```python
from build123d import *

# Parameters (mm, degrees)
SKETCH1_W           = 120
SKETCH1_H           = 31
BOSS_EXTRUDE1_DEPTH = 10
SKETCH4_R           = 3
BOSS_EXTRUDE2_DEPTH = 30
FILLET1_R           = 2


with BuildPart() as part:
    # Sketch1 → Boss-Extrude1 (new body, symmetric)
    with BuildSketch(Plane(origin=(0, 0, 0), x_dir=(1, 0, 0), z_dir=(0, 1, 0))):
        Rectangle(SKETCH1_W, SKETCH1_H)
    extrude(amount=BOSS_EXTRUDE1_DEPTH, both=True)

    # Sketch4 → Boss-Extrude2 (add)
    with BuildSketch(Plane(origin=(-32.75, 0, -32.75), x_dir=(0.707106781, 0, -0.707106781), z_dir=(0.707106781, 0, 0.707106781))):
        with Locations((-26.466251763, 4)):
            Circle(SKETCH4_R)
        with Locations((-26.466251763, -4)):
            Circle(SKETCH4_R)
    extrude(amount=-BOSS_EXTRUDE2_DEPTH)

    # Fillet1
    fillet1_edges = [part.edges().sort_by_distance(p)[0] for p in [
        (-60, 10, 0),
        (0, 10, 15.5),
        (60, 10, 0),
        (0, -10, 15.5),
        (-60, -10, 0),
        (0, -10, -15.5),
        (60, -10, 0),
        (60, 0, 15.5),
        (-60, 0, 15.5),
        (-60, 0, -15.5),
        (60, 0, -15.5),
        (0, 10, -15.5),
    ]]
    fillet(fillet1_edges, radius=FILLET1_R)


solid = part.part
```
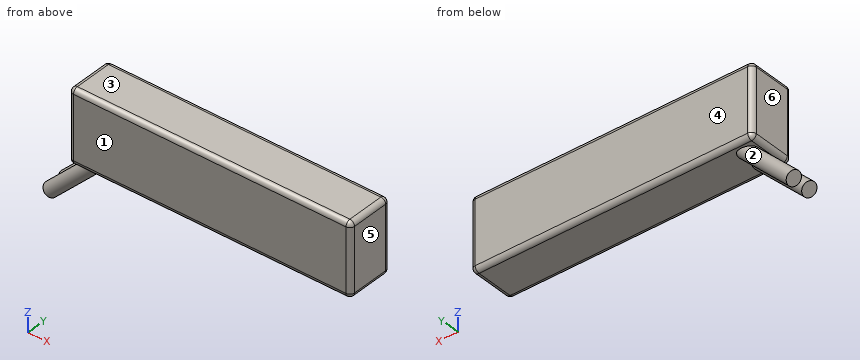
Input: part model. Units: mm. Frame: model coordinates. Face numbers are marked on the shaded views. A direction names the side the tool comes from. Give positions to 0.01 mm unless a question says otherwise; leave off trailing zeros. Order: outer loops, then holes, each group sorted by start corner. A loop starts at its lowest first (then second) coordinate and runs counter-clockwise, first axis right, second up.
1. Line query: probe 1 along X at (y, z) = (-8, -8); probe 2 along Z at (x, y) = (43.5, -4.25); probe 3 along Z at (x, y) = (-52, 4.5). Output: solid intervals per line, ascending.
Computed:
probe 1: x = -60 to 60
probe 2: z = -15.5 to 15.5
probe 3: z = -18.75 to 15.5
2. Draft query along Y for the marked faces 1, 2, 3 and 4. Return one class per face: released by +Y, released by -Y, zero draft, split by the parting line, or undercut.
Computed:
face 1: released by -Y
face 2: undercut
face 3: zero draft
face 4: released by +Y
3. Cut plane A-A (x = 15). Return loops of the section in (y, z).
Computed:
outline: (-10, -13.5) arc R2 ccw to (-8, -15.5) - (8, -15.5) arc R2 ccw to (10, -13.5) - (10, 13.5) arc R2 ccw to (8, 15.5) - (-8, 15.5) arc R2 ccw to (-10, 13.5) - close
4. Set-up query: the marked faces 5 and 6. Return all of +Z, -Z, +X, -X, +Y, -Y with unobstructed straight access to the full face (end or side cutting, diameter ignored); none if empty.
Computed:
face 5: +Z, -Z, +X, +Y, -Y
face 6: +Z, -X, +Y, -Y
5. Pin query (flat end, axial travel): pin 1 Ø10 at (y, z) = (-7.5, 2.5) entering from -X; pin 2 Ø12 at (y, z) = (-4.5, -24.5) entering from +X; pin 3 Ø4 at (x, y) = (35, 3) entering from -Z; pin 4 Ø8 at (x, y) = (-61, -1) entering from +Z. Return the tip coordinate at first contact, or that it passes through.
Computed:
pin 1: stops at x = -60
pin 2: stops at x = -51.7
pin 3: stops at z = -15.5
pin 4: stops at z = 15.5
6. Cut plane B-B (z = 11). Return loops of the section in (x, y).
Computed:
outline: (-60, -8) arc R2 ccw to (-58, -10) - (58, -10) arc R2 ccw to (60, -8) - (60, 8) arc R2 ccw to (58, 10) - (-58, 10) arc R2 ccw to (-60, 8) - close
